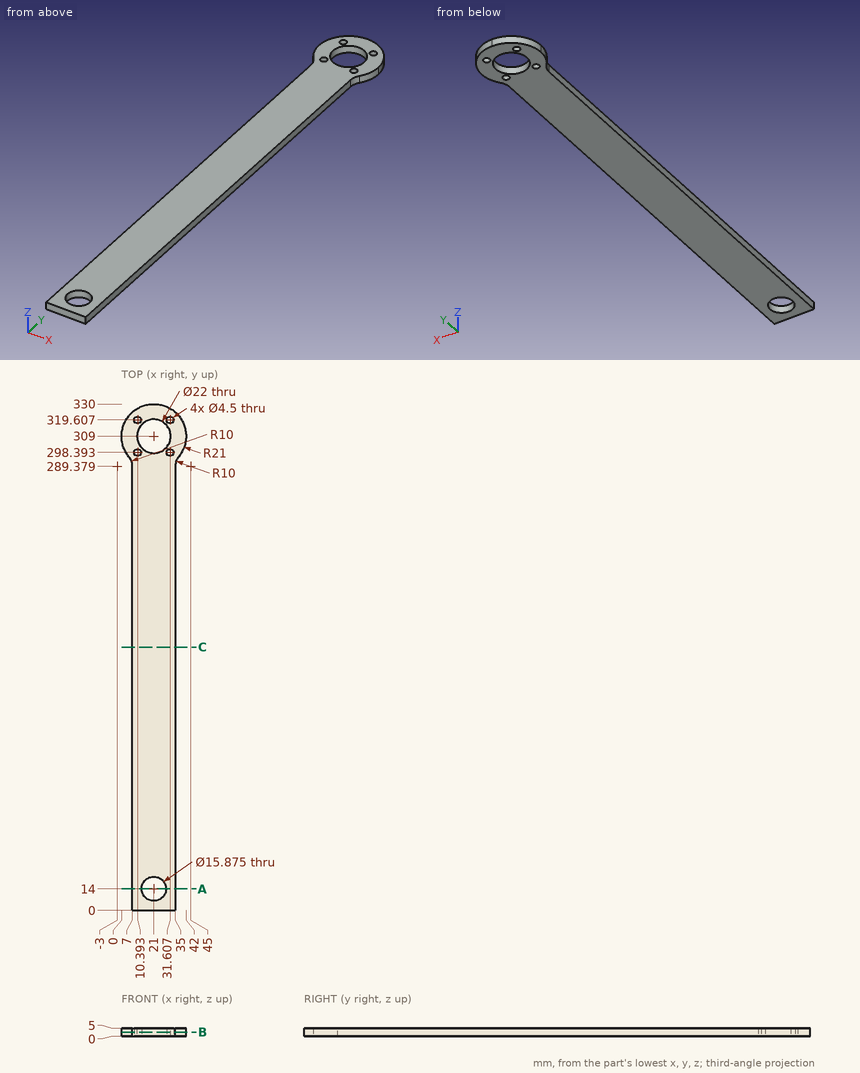
For this review, use the dimensioned drawing (mm, ordinates from the lowest corner) and the shaded views. Coordinates: 2 decimals unless noted, no trailing zeros. Loops run counter-clockwise (first coordinate to the right, second up) from the corner with the lowest first, then second, coordinate; pieces in that order, holes last. Notation, with made-up numbers: (46, 30.5) - (59, 30.5) arc R25 ccw to (59, 42.5) - close; hole circle Ø9 at (-9, -16). An arc over 180 degrees is marked (long way). Use CSV: the item, a comma, the result in double quotes. Start each with the question number.
1) Consider section A-A on y = 14. Write out the cut boundary in (x, z).
2) Consider section B-B on z = 2.55. Give the number of separate pieces and of enclosed holes in the cut face, then the cut area to 3 significant figures.
3) Consider section C-C on y = 171.5. Write out the cut boundary in (x, z), then the cut area to 3 significant figures.
4) For pin 1 Ø18.5 at (x, y) = (21, 14) entering from +Z; pin 2 Ø4 at (x, y) = (10.39, 298.39) entering from +Z; pin 3 Ø1.5 at (y, z) = (74.5, 1.5) entering from +X; pin 4 Ø1.5 at (y, z) = (115, 2) entering from -X, all flat-tipped, find the tip position at first contact; note any pin that passes through.
5) Wall thickness on L1, parallel to Y at x = 22, z = 3 (1 decimal); L2, parallel to Y at x = 26, z = 1.3 (1 decimal); L3, parallel to X at y = 161, z = 3.75: over which ranges is each line inside the solid? List them lowest first. Write a range as from..to.
Geometry says:
1,outline,"(7, 0) - (13.06, 0) - (13.06, 5) - (7, 5) - close; (28.94, 0) - (35, 0) - (35, 5) - (28.94, 5) - close"
2,separate pieces,"1"
2,enclosed holes,"6"
2,area,"8,860 mm^2"
3,outline,"(7, 0) - (35, 0) - (35, 5) - (7, 5) - close"
3,area,"140 mm^2"
4,pin 1,"z = 5"
4,pin 2,"through"
4,pin 3,"x = 35"
4,pin 4,"x = 7"
5,L1,"0..6.1, 21.9..298, 320..330"
5,L2,"0..7.8, 20.2..299.2, 318.8..329.4"
5,L3,"7..35"
